Read the model definition and answer for the solid it produces. Units are mm, in the model's axes. Face numbers are marked on the shaded views. Coordinates: 2 decimals unless noted, no trailing zeros. Order: outer loops, then holes, each group sorted by start corner. A loop starts at its lowest first (then second) coordinate and runs counter-clockwise, first axis right, second up. Notation, with made-up numbers: (-5.5, -16.5) -> (5.5, -16.5) arc R27 cw to (5.5, -0.5) -> close; hole circle Ø4 at (81, -21). An arc over 180 degrees is marked (long way). Return JSON: item names as keys, results as strings. Group by question number.
```python
from build123d import *

# Parameters (mm, degrees)
SKETCH1_R           = 34.798
BOSS_EXTRUDE1_DEPTH = 6.35
FILLET1_R           = 2.54
SKETCH2_R           = 5.08
CUT_EXTRUDE1_DEPTH  = 6.35
SKETCH3_R           = 2.54
CUT_EXTRUDE2_DEPTH  = 19.05
CIRPATTERN1_COUNT   = 8


with BuildPart() as part:
    # Sketch1 → Boss-Extrude1 (new body)
    with BuildSketch(Plane(origin=(0, 0, 0), x_dir=(0, 0, -1), z_dir=(1, 0, 0))):
        Circle(SKETCH1_R)
    extrude(amount=BOSS_EXTRUDE1_DEPTH)

    # Fillet1
    fillet1_edges = [part.edges().sort_by_distance(p)[0] for p in [
        (6.35, 0, 34.798),
    ]]
    fillet(fillet1_edges, radius=FILLET1_R)

    # Sketch2 → Cut-Extrude1 (cut)
    with BuildSketch(Plane(origin=(6.35, 0, 0), x_dir=(0, 0, -1), z_dir=(1, 0, 0))):
        Circle(SKETCH2_R)
    extrude(amount=-CUT_EXTRUDE1_DEPTH, mode=Mode.SUBTRACT)

    # Sketch3 → Cut-Extrude2 (cut)
    with BuildSketch(Plane(origin=(6.35, 0, 0), x_dir=(0, 0, -1), z_dir=(1, 0, 0))):
        with Locations((22.543897228, 0)):
            Circle(SKETCH3_R)
    cut_extrude2 = extrude(amount=-CUT_EXTRUDE2_DEPTH, mode=Mode.SUBTRACT)

    # CirPattern1: Cut-Extrude2 ×8 about axis
    cirpattern1_axis = Axis((0, 0, 0), (1, 0, 0))
    for i in range(1, CIRPATTERN1_COUNT):
        add(cut_extrude2.rotate(cirpattern1_axis, i * 360 / CIRPATTERN1_COUNT), mode=Mode.SUBTRACT)


solid = part.part
```
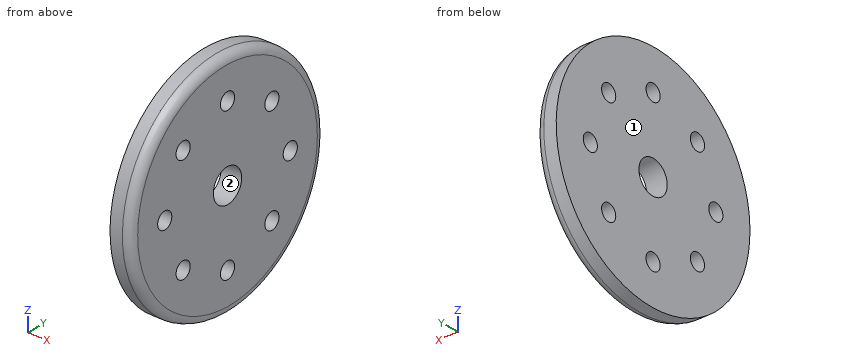
1. For a pull along Y with two mould halves and no side action, classify the marked faces 1 and 2 as released by +Y, released by -Y, zero draft, split by the parting line, or undercut.
2. Find section C-C on x = 1.5. Give the number of separate pieces and of enclosed holes in the cut face, and give its area (3 significant figures).
3. Find section A-A on z = 0. Determine the outline of the cut face in (x, y).
4. Straight lines are drawn through the part: L1, parallel to Y at x = 2, z = 16.5; L2, parallel to Z at x = 4.75, y = 16; L3, parallel to Y at x = 5.25, z = 15.5. For each, find the intervals that lie inside material, in ascending order.
5. Given pin 1 (6 mm diameter, centred on y = 0, z = -22.54, fed in from +X); pin 2 (1.5 mm diameter, centred on x = 1.5, z = 27, fed in from +Y); pin 3 (2 mm diameter, centred on x = 4, y = -22, fed in from -Z); pin 4 (1 mm diameter, centred on x = 2, y = -9.5, fed in from +Z), each flat-ended and moving along its own axis, determine where each tip first touches the part or whether it passes through.
Result:
{
 "1": {"face 1": "zero draft", "face 2": "undercut"},
 "2": {"separate pieces": "1", "enclosed holes": "9", "area": "3,560 mm^2"},
 "3": {"outline": "(0, -34.8) -> (3.81, -34.8) arc R2.54 ccw to (6.35, -32.26) -> (6.35, -25.08) -> (0, -25.08) -> close; (0, -20) -> (6.35, -20) -> (6.35, -5.08) -> (0, -5.08) -> close; (0, 5.08) -> (6.35, 5.08) -> (6.35, 20) -> (0, 20) -> close; (0, 25.08) -> (6.35, 25.08) -> (6.35, 32.26) arc R2.54 ccw to (3.81, 34.8) -> (0, 34.8) -> close"},
 "4": {"L1": "-30.64 to -18.42, -13.46 to 13.46, 18.42 to 30.64", "L2": "-30.7 to -18.48, -13.4 to 13.4, 18.48 to 30.7", "L3": "-30.65 to -18.44, -13.44 to 13.44, 18.44 to 30.65"},
 "5": {"pin 1": "x = 6.35", "pin 2": "y = 22.84", "pin 3": "z = -27.74", "pin 4": "z = 33.61"}
}
